Verification items for the finished model (mm, model axes). Face numbers are marked on the shaded views. A direction names the side the tool comes from. Coordinates: 2 decimals unless noted, no trailing zeros. Order: outer loops, then holes, each group sorted by start corner. A loop starts at its lowest first (then second) coordinate and runs counter-clockwise, first axis right, second up. Notation, with made-up numbers: M 28.5,62 L 48.5,62 A30 cw 48.5,98 Z; hole C 43.5,-3 d8. An arc over 180 degrees is marked long. Return JSON: item names as keys, results as strings. Group by question number.
1. Material ranges on line 1 along X through (y, z) = (13.9, 9); line 2 along Z through (x, y) = (11.5, 7); line 3 along Y through (x, z) = (11.15, 1.5), recorded low to high.
2. Mould release check, pull along X, two halves, no side actions. Record for the marked faces 4, 5, 6 and 7: +X half, -X half, draft (parallel to the pull), parting line (faces both ways), or undercut.
3. Gauge pin test, flat ends, axial feed: pin 1 (1 mm diameter, centred on y = -7, z = 8, fed in from -X); pin 2 (6 mm diameter, centred on y = 9, z = 5, fed in from +X); pin 3 (2.5 mm diameter, centred on x = -3, z = 9, fed in from -Y). Record the tip position at first contact, or that the pin passes through.
4. Section check C-C, the plane z = 9.5. Record the cut outline in (x, y), plus the area to 3 significant figures.
5. Section check D-D, the plane y = -8.75. Record the cut outline in (x, z).
6. Section check A-A, the plane x = -3. Record the cut outline in (y, z), plus the area to 3 significant figures.
7. Set-up check for the marked faces 1, 2 and 3: record each of +Z, -Z, +X, -X, +Y, -Y from which the full face is reachable in a straight line by a thin tool's end or side.
8. Section check B-B, the plane z = 1.5. Record the cut outline in (x, y).
```python
from build123d import *

# Parameters (mm, degrees)
SKETCH1_W           = 24
SKETCH1_H           = 29
SKETCH1_W_2         = 21
SKETCH1_H_2         = 26
BOSS_EXTRUDE1_DEPTH = 12
SKETCH2_W           = 21
SKETCH2_H           = 12
CUT_EXTRUDE1_DEPTH  = 33.314857264
SKETCH4_W           = 12
SKETCH4_H           = 22.5
CUT_EXTRUDE2_DEPTH  = 12
SKETCH5_R           = 0.5
CUT_EXTRUDE3_DEPTH  = 12
SKETCH6_R           = 0.5
CUT_EXTRUDE4_DEPTH  = 12
SKETCH7_R           = 2
BOSS_EXTRUDE2_DEPTH = 4
SKETCH9_R           = 1
CUT_EXTRUDE5_DEPTH  = 10


with BuildPart() as part:
    # Sketch1 → Boss-Extrude1 (new body)
    with BuildSketch(Plane.XY):
        Rectangle(SKETCH1_W, SKETCH1_H)
        Rectangle(SKETCH1_W_2, SKETCH1_H_2, mode=Mode.SUBTRACT)
    extrude(amount=BOSS_EXTRUDE1_DEPTH)

    # Sketch2 → Cut-Extrude1 (cut, through all)
    with BuildSketch(Plane(origin=(0, -13, 0), x_dir=(1, 0, 0), z_dir=(0, 1, 0))):
        with Locations((0, -6)):
            Rectangle(SKETCH2_W, SKETCH2_H)
    extrude(amount=-CUT_EXTRUDE1_DEPTH, mode=Mode.SUBTRACT)

    # Sketch4 → Cut-Extrude2 (cut)
    with BuildSketch(Plane.ZY.offset(12)):
        with Locations((6, -3.25)):
            Rectangle(SKETCH4_W, SKETCH4_H)
    extrude(amount=-CUT_EXTRUDE2_DEPTH, mode=Mode.SUBTRACT)

    # Sketch5 → Cut-Extrude3 (cut)
    with BuildSketch(Plane(origin=(12, 0, 0), x_dir=(0, 0, -1), z_dir=(1, 0, 0))):
        with Locations(Location((-10.5, -13, 0), (0, 0, 90))):
            Circle(SKETCH5_R)
        with Locations(Location((-1.5, -13, 0), (0, 0, 270))):
            Circle(SKETCH5_R)
        with Locations(Location((-10.5, 7, 0), (0, 0, 90))):
            Circle(SKETCH5_R)
        with Locations(Location((-1.5, 7, 0), (0, 0, 270))):
            Circle(SKETCH5_R)
    extrude(amount=-CUT_EXTRUDE3_DEPTH, mode=Mode.SUBTRACT)

    # Sketch6 → Cut-Extrude4 (cut)
    with BuildSketch(Plane.ZY.offset(12)):
        with Locations(Location((9.5, 10.5, 0), (0, 0, 270))):
            Circle(SKETCH6_R)
        with Locations(Location((2.5, 10.5, 0), (0, 0, 90))):
            Circle(SKETCH6_R)
    extrude(amount=-CUT_EXTRUDE4_DEPTH, mode=Mode.SUBTRACT)

    # Sketch7 → Boss-Extrude2 (add)
    with BuildSketch(Plane(origin=(12, 0, 0), x_dir=(0, 0, -1), z_dir=(1, 0, 0))):
        with Locations(Location((-6, -8.5, 0), (0, 0, 270))):
            Circle(SKETCH7_R)
    extrude(amount=BOSS_EXTRUDE2_DEPTH)

    # Sketch9 → Cut-Extrude5 (cut)
    with BuildSketch(Plane(origin=(0, 14.5, 0), x_dir=(1, 0, 0), z_dir=(0, 1, 0))):
        with Locations(Location((6, -3, 0), (0, 0, 270))):
            Circle(SKETCH9_R)
        with Locations(Location((6, -9, 0), (0, 0, 90))):
            Circle(SKETCH9_R)
        with Locations(Location((-3, -3, 0), (0, 0, 270))):
            Circle(SKETCH9_R)
        with Locations(Location((-3, -9, 0), (0, 0, 90))):
            Circle(SKETCH9_R)
    extrude(amount=-CUT_EXTRUDE5_DEPTH, mode=Mode.SUBTRACT)


solid = part.part
```
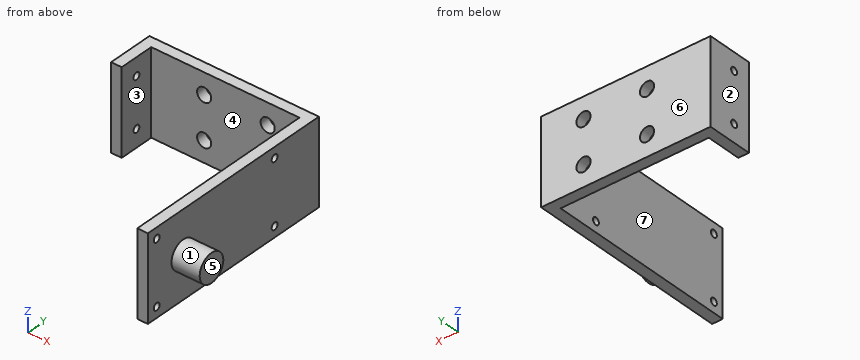
Answers follow:
{
 "1": {"line 1": "-12 to -4, -2 to 5, 7 to 12", "line 2": "0 to 1, 2 to 10, 11 to 12", "line 3": "-14.5 to -13.5, -12.5 to 6.5, 7.5 to 14.5"},
 "2": {"face 4": "undercut", "face 5": "+X half", "face 6": "draft", "face 7": "undercut"},
 "3": {"pin 1": "x = 10.5", "pin 2": "x = 12", "pin 3": "y = 13"},
 "4": {"outline": "M -12,8 L -10.5,8 L -10.5,10 L -12,10 Z; M -12,11 L -10.5,11 L -10.5,13 L -3.87,13 L -3.87,14.5 L -12,14.5 Z; M -2.13,13 L 5.13,13 L 5.13,14.5 L -2.13,14.5 Z; M 6.87,13 L 10.5,13 L 10.5,-14.5 L 12,-14.5 L 12,14.5 L 6.87,14.5 Z", "area": "78.1 mm^2"},
 "5": {"outline": "M 10.5,0 L 12,0 L 12,4.02 L 16,4.02 L 16,7.98 L 12,7.98 L 12,12 L 10.5,12 Z"},
 "6": {"outline": "M 13,0 L 14.5,0 L 14.5,2 L 13,2 Z; M 13,4 L 14.5,4 L 14.5,8 L 13,8 Z; M 13,10 L 14.5,10 L 14.5,12 L 13,12 Z", "area": "12.0 mm^2"},
 "7": {"face 1": "+X", "face 2": "+Z, -Z, -X, +Y, -Y", "face 3": "+Z, -Z, -Y"},
 "8": {"outline": "M -12,8 L -10.5,8 L -10.5,13 L 10.5,13 L 10.5,7.5 L 12,7.5 L 12,14.5 L -12,14.5 Z; M 10.5,-14.5 L 12,-14.5 L 12,-13.5 L 10.5,-13.5 Z; M 10.5,-12.5 L 12,-12.5 L 12,6.5 L 10.5,6.5 Z"}
}
